Input: dimensioned drawing with shaded views. Units: mm. Origin: part minimum x, y, z. A direction names the side the tool comes from. Coordinates: 2 decimals unless noted, no trailing zeros. Write each loop counter-clockwise with the first axis right and the second up, starting at its lowest first coordinate (ties: lowest second). Pieces come first, ordered by that corner, then holes. Notation, with made-up numbers: (16, -18.75) -> (61, -18.75) arc R32 cw to (61, 15.25) -> close; hole circle Ø6 at (31.25, 84). An arc over 180 degrees is marked (long way). One line per item, written item: value. Start each with the question number.
1. Line query: line 1 (Z direction, x = 48.5, y = 4.5); line 2 (X direction, y = 5, z = 43); line 3 (Y direction, x = 24, z = 42). Output: solid intervals per line, ascending.
2. Section query B-B, the plane y = 13.75. Output: boundary loops of the cut face in (x, z).
3. Mould query, pull axis X, two halves, no side actions, for the marked faces 4, 5 and 6. Classes: released by +X, released by -X, zero draft, split by the parting line, or undercut.
4. Section query A-A, the plane z = 32. Output: boundary loops of the cut face in (x, y).
5. Access query for the marked faces 1, 2 and 3. Directions: +Z, -Z, +X, -X, +Y, -Y. A direction counts if a zero-diameter tool reaches every point of the face in a straight line with its end or side. Return the directions, or none.
6. Section query C-C, the plane x = 21.5. Output: boundary loops of the cut face in (y, z).
7. First-contact query: P1, Ø1.5, axis at x = 12.5, z = 8, coming from the -Y side. Flat tip, straight axial feed; report the tip coordinate or a pass-through.
8. Section query D-D, the plane x = 8. Output: boundary loops of the cut face in (y, z), and give its area (3 significant figures).
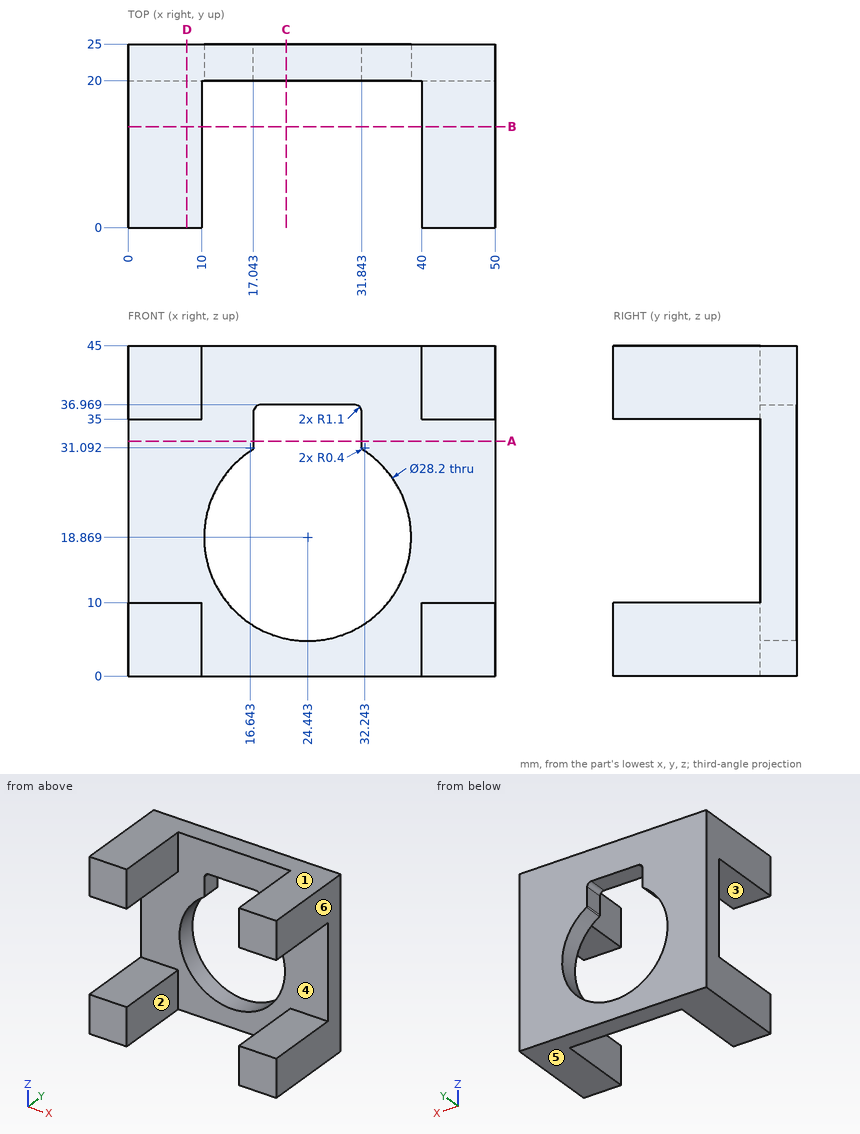
Computed values:
1. line 1: z = 0 to 10, 35 to 45
1. line 2: x = 0 to 10, 40 to 50
1. line 3: y = 20 to 25
2. outline: (0, 0) -> (10, 0) -> (10, 10) -> (0, 10) -> close; (0, 35) -> (10, 35) -> (10, 45) -> (0, 45) -> close; (40, 0) -> (50, 0) -> (50, 10) -> (40, 10) -> close; (40, 35) -> (50, 35) -> (50, 45) -> (40, 45) -> close
3. face 4: undercut
3. face 5: zero draft
3. face 6: released by +X
4. outline: (0, 20) -> (17.04, 20) -> (17.04, 25) -> (0, 25) -> close; (31.84, 20) -> (50, 20) -> (50, 25) -> (31.84, 25) -> close
5. face 1: +Z, +X, -X, +Y, -Y
5. face 2: +Z, -Z, -Y
5. face 3: +X, -X, -Y
6. outline: (20, 0) -> (25, 0) -> (25, 5.08) -> (20, 5.08) -> close; (20, 36.97) -> (25, 36.97) -> (25, 45) -> (20, 45) -> close
7. P1: stops at y = 20
8. outline: (0, 0) -> (25, 0) -> (25, 45) -> (0, 45) -> (0, 35) -> (20, 35) -> (20, 10) -> (0, 10) -> close
8. area: 625 mm²
